Here's the drawing with two shaded views (mm, measured from the low corner). I have some questions. Give positions to 0.01 mm unless a question says otherwise; leave off trailing zeros. Loops run counter-clockwise (first coordinate to the right, second up) from the corner with the lowest first, then second, coordinate; pieces in that order, holes last. Notation, with made-up numbers: (84, 88) - (105, 88) arc R22 ccw to (105, 112) - close; hole circle Ø6 at (66, 7). An arc over 180 degrees is marked (long way). Answer as a JSON object with one key per item and string values. Group by question number.
Item 1: Please list where these lines run through material, in increasing order: L1, parallel to Y at x = 49.5, z = 2.95; L2, parallel to X at y = 86.5, z = 3.85.
Item 2: Suppose I cut it at B-B on z = 3.45. Write out the boundary of the cut face in (x, y), and give its area (3 significant figures).
Item 3: Will this pin go through, and if not, where does the flat tip stop? pin 1 (1.5 mm diameter, centred on y = 111.5, z = 1, fed in from -X).
Item 4: Suppose I cut it at A-A on x = 70.5. Write out the boundary of the cut face in (y, z), and give its area (3 significant figures).
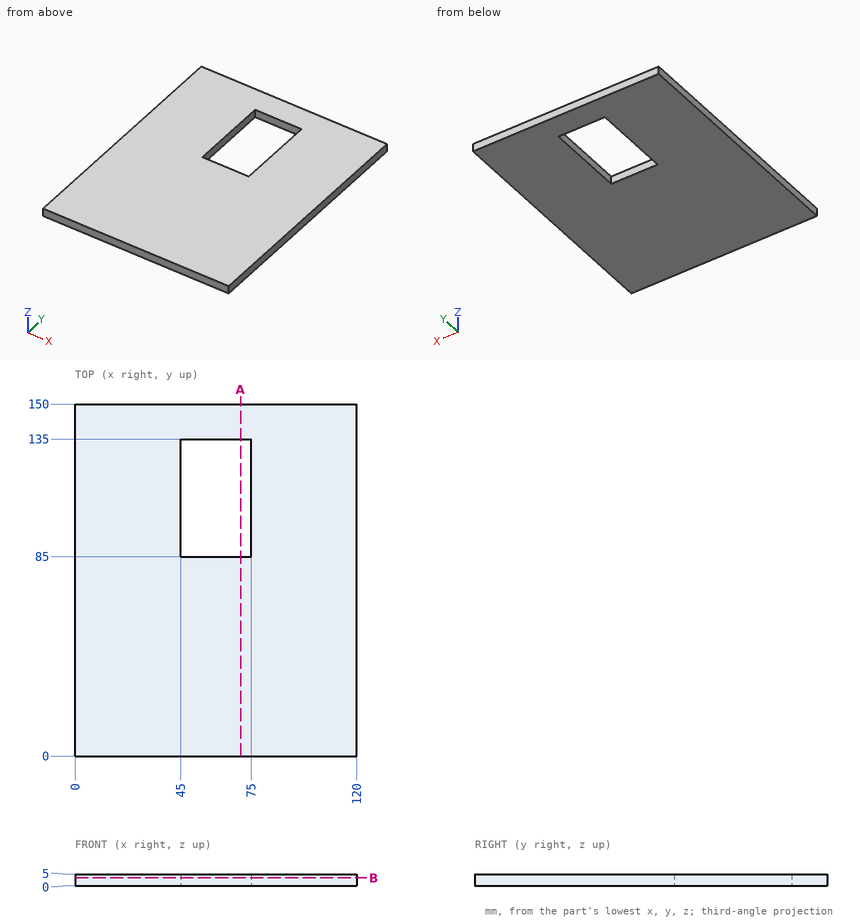
Worked out:
{
 "1": {"L1": "y = 0 to 85, 135 to 150", "L2": "x = 0 to 45, 75 to 120"},
 "2": {"outline": "(0, 0) - (120, 0) - (120, 150) - (0, 150) - close; hole (45, 85) - (75, 85) - (75, 135) - (45, 135) - close", "area": "16,500 mm2"},
 "3": {"pin 1": "stops at x = 0"},
 "4": {"outline": "(0, 0) - (85, 0) - (85, 5) - (0, 5) - close; (135, 0) - (150, 0) - (150, 5) - (135, 5) - close", "area": "500 mm2"}
}
